Autodesk Inventor part; units mm, degrees
ref_plane "YZ Plane" through (0, 0, 0) normal (1, 0, 0) x (0, 1, 0)
ref_plane "XZ Plane" through (0, 0, 0) normal (0, 1, 0) x (-1, 0, 0)
ref_plane "XY Plane" through (0, 0, 0) normal (0, 0, 1) x (1, 0, 0)
sketch "Sketch1" plane through (0, 0, 0) normal (0, 1, 0) x (-1, 0, 0)
  line L0 (-17.975, -21.15) -> (17.975, -21.15)
  line L1 (21.15, -17.975) -> (21.15, 17.975)
  line L2 (17.975, 21.15) -> (-17.975, 21.15)
  line L3 (-21.15, 17.975) -> (-21.15, -17.975)
  line L4 (-21.15, -21.15) -> (21.15, 21.15) construction
  line L5 (21.15, -21.15) -> (-21.15, 21.15) construction
  line L6 (17.975, 21.15) -> (21.15, 17.975)
  line L7 (-17.975, 21.15) -> (-21.15, 17.975)
  line L8 (-21.15, -17.975) -> (-17.975, -21.15)
  line L9 (17.975, -21.15) -> (21.15, -17.975)
  point P0 (0, 0)
  dimension "d0" = 42.3
  dimension "d1" = 42.3
  dimension "d2" = 3.175
  dimension "d3" = 3.175
  dimension "d4" = 3.175
  dimension "d5" = 3.175
  dimension "d6" = 3.175
  dimension "d7" = 3.175
  dimension "d8" = 3.175
  dimension "d9" = 3.175
extrude "Extrusion1" add sketch "Sketch1" along normal blind 34
sketch "Sketch2" plane through (0, 34, 0) normal (0, 1, 0) x (1, 0, 0)
  circle A0 centre (0, 0) radius 11
  dimension "d12" = 22
extrude "Extrusion2" add sketch "Sketch2" along normal blind 2
sketch "Sketch3" plane through (0, 36, 0) normal (0, 1, 0) x (1, 0, 0)
  circle A0 centre (0, 0) radius 2.5
  dimension "d15" = 5
extrude "Extrusion3" add sketch "Sketch3" along normal blind 22
sketch "Sketch4" plane through (0, 34, 0) normal (0, 1, 0) x (1, 0, 0)
  line L0 (89.125, 0) -> (-55.025, 0)
  line L1 (0, 94.2917) -> (0, -108.2417)
  point P0 (0, 0)
  point P1 (15.5, 15.5)
  point P2 (15.5, -15.5)
  point P3 (-15.5, 15.5)
  point P4 (-15.5, -15.5)
  dimension "d18" = 31
  dimension "d19" = 31
hole "Hole1" at (15.5, 34, -15.5) at (15.5, 34, 15.5) at (-15.5, 34, -15.5) at (-15.5, 34, 15.5) direction (0, -1, 0) diameter 2.4638 depth 5 tip angle 118
equation "\"d1\" = d0"
equation "\"d3\" = d2"
equation "\"d4\" = d2"
equation "\"d5\" = d4"
equation "\"d6\" = d2"
equation "\"d7\" = d6"
equation "\"d8\" = d2"
equation "\"d9\" = d8"
properties part number "Stepper_Motor"
Input: part model. Units: mm. Frame: model coordinates. A direction names the side the tool comes from. Coordinates: 2 decimals unless noted, no trailing zeros. Order: outer loops, then holes, each group sorted by start corner. A loop starts at its lowest first (then second) coordinate and runs counter-clockwise, first axis right, second up. Notation, with made-up numbers: M 64,10.5 L 79,10.5 A21 ccw 79,29.5 Z; hole C 72.5,70 d3. An arc over 180 degrees is marked long. Write item = value, one per line. Start each with the question number.
(1) Section D-D on x = -6.5. Output: boundary loops of the cut face in (y, z), and give its area (3 significant figures).
(2) Section A-A on z = 0. Output: boundary loops of the cut face in (x, y), and give its area (3 significant figures).
(3) Reachability of faces 1 (the flat face through (-19.54, 16.762, -19.585)), 2 (the cylindrical face through (-2.38, 34.99, -10.74)) from +Z, -Z, +X, -X, +Y, -Y: full face, straight path, thin tool, end or side. Return the list, or none.
(4) Section C-C on y = 48. Output: boundary loops of the cut face in (x, z).
(5) Pull-direction query (X, two-part tool) for faces 3 (the cylindrical face through (-16.54, 31.46, -14.84)), 4 (the flat face through (10, 34, -9)), 5 (the flat face through (-19.54, 16.762, 19.585)); classes: released by +X, released by -X, zero draft, split by the parting line, or undercut.
(6) Line query: line 1 along Z through (x, y) = (-15.5, 31.9); line 2 along Z through (x, y) = (15, 31). Output: solid intervals per line, ascending. Write a range as [from, to].
(7) First-contact query: P1, Ø6, axis at x = -16, z = 10.5, coming from the +Y side; P2, Ø1.5, axis at x = 4, z = 1, coming from the +Y side. Flat tips, straight axial feed; report the tip coordinate or a pass-through.
(8) Section B-B on x = 0. Output: boundary loops of the cut face in (y, z).
Result set:
q1.outline = M 0,-21.15 L 34,-21.15 L 34,-8.87 L 36,-8.87 L 36,8.87 L 34,8.87 L 34,21.15 L 0,21.15 Z
q1.area = 1,470 mm²
q2.outline = M -21.15,0 L 21.15,0 L 21.15,34 L 11,34 L 11,36 L 2.5,36 L 2.5,58 L -2.5,58 L -2.5,36 L -11,36 L -11,34 L -21.15,34 Z
q2.area = 1,590 mm²
q3.face_1 = -Z, -X, +Y, -Y
q3.face_2 = +Y
q4.outline = C 0,0 d5
q5.face_3 = undercut
q5.face_4 = zero draft
q5.face_5 = released by -X
q6.line_1 = [-21.15, -16.73], [-14.27, 14.27], [16.73, 21.15]
q6.line_2 = [-21.15, -16.63], [-14.37, 14.37], [16.63, 21.15]
q7.P1 = 34
q7.P2 = 36
q8.outline = M 0,-21.15 L 34,-21.15 L 34,-11 L 36,-11 L 36,-2.5 L 58,-2.5 L 58,2.5 L 36,2.5 L 36,11 L 34,11 L 34,21.15 L 0,21.15 Z
